Can you work these out from the model? Positions are in its coordinate system, mm. A direction names the side the tool comes from. Give positions to 0.01 mm unless a question says otherwise; leave off trailing zeros. Loops run counter-clockwise (first coordinate to the right, second up) from the corner with the lowest first, then second, coordinate; pieces in that order, holes last. Notation, with made-up numbers: (58, 79.5) - (79, 79.5) arc R13 ccw to (79, 83.5) - close; hole circle Ø8 at (88.5, 71). An arc over 180 degrees is marked (long way). Answer as a JSON object with one key per item and string values. Group by question number.
Item 1: Suppose I cut it at A-A on z = 77.5. Write out the boundary of the cut face in (x, y).
Item 2: Thinking about a two-plate mould opening in X: for faces 1 (the flat face through (-1, 1, 0)), 2 (the flat face through (27.978, -37, 5)), 3 (the flat face through (20, -37, 13)), 4 (the flat face through (-44, -1, 8)), which applies, pulls with the +X half, pulls with the -X half, needs draft (parallel to the pull), parting line crosses it, or undercut?
Item 3: Which directions (+Z, -Z, +X, -X, +Y, -Y) give clear straight access to the entire face, cutting with the end or side of a thin tool? Please do faces 5 (the cylindrical face through (-42, 14, 13)), 6 (the flat face through (21, -48.582, 5)), 7 (the flat face through (0, -58, 150)).
Item 4: Please list where these lines run through material, in increasing order: L1, parallel to Z at x = -6, y = 66; L2, parallel to X at y = -34, z = 49.5; L3, parallel to Y at x = -40, z = 77.
Item 5: Will these pins go through, and if not, where does the flat tip stop? pin 1 (1.5 mm diameter, centred on x = 22, z = -2, fed in from -Y); pin 2 (3 mm diameter, centred on x = -26.5, y = 0.5, fed in from -Z); pin 3 (8 mm diameter, centred on x = 17, y = -31.5, fed in from -Z).
Item 6: Suppose I cut it at B-B on y = 0. Write out the boundary of the cut face in (x, z).
Item 7: Suppose I cut it at C-C on x = 0. Write out the boundary of the cut face in (y, z), and give its area (3 significant figures).
Item 8: Suppose I cut it at D-D on x = -17. Write out the boundary of the cut face in (y, z), and give its area (3 significant figures).
from build123d import *

# Parameters (mm, degrees)
SKETCH_W        = 88
SKETCH_H        = 160
PAD_DEPTH       = 155
SKETCH001_R     = 66
POCKET_DEPTH    = 5
POCKET001_DEPTH = 5
SKETCH003_W     = 24
SKETCH003_H     = 31
PAD001_DEPTH    = 3
SKETCH004_W     = 16
SKETCH004_H     = 23
POCKET002_DEPTH = 16
CHAMFER_SIZE    = 3


with BuildPart() as part:
    # Sketch (on XY_Plane of Origin) → Pad (new body)
    with BuildSketch(Plane.XY):
        Rectangle(SKETCH_W, SKETCH_H)
    extrude(amount=PAD_DEPTH)

    # Sketch001 (on Face4 of Pad) → Pocket (cut)
    with BuildSketch(Plane(origin=(-44, 0, 0), x_dir=(0, -1, 0), z_dir=(-1, 0, 0))):
        with Locations((0, 77.5)):
            Circle(SKETCH001_R)
    extrude(amount=-POCKET_DEPTH, mode=Mode.SUBTRACT)

    # Sketch002 (on Face5 of Pocket) → Pocket001 (cut)
    with BuildSketch(Plane.XY.offset(155)):
        with BuildLine():
            ThreePointArc((20, -56.995285), (0, -36.995285), (-20, -56.995285))
            Line((-20, -56.995285), (-20, -80))
            Line((-20, -80), (20, -80))
            Line((20, -56.995285), (20, -80))
        make_face()
    extrude(amount=-POCKET001_DEPTH, mode=Mode.SUBTRACT)

    # Sketch003 (on Face2 of Pocket001) → Pad001 (join)
    with BuildSketch(Plane(origin=(0, 0, 0), x_dir=(1, 0, 0), z_dir=(0, 0, -1))):
        with Locations((19.978081, 37.081905)):
            Rectangle(SKETCH003_W, SKETCH003_H)
    extrude(amount=PAD001_DEPTH)

    # Sketch004 (on Face16 of Pad001) → Pocket002 (cut)
    with BuildSketch(Plane(origin=(0, 0, -3), x_dir=(1, 0, 0), z_dir=(0, 0, -1))):
        with Locations((19.978081, 37.081905)):
            Rectangle(SKETCH004_W, SKETCH004_H)
    extrude(amount=-POCKET002_DEPTH, mode=Mode.SUBTRACT)

    # Chamfer
    chamfer_edges = [part.edges().sort_by_distance(p)[0] for p in [
        (11.978081, -25.581905, 5),
        (11.978081, -48.581905, 5),
    ]]
    chamfer(chamfer_edges, length=CHAMFER_SIZE)


solid = part.part
Worked out:
{
 "1": {"outline": "(-44, -80) - (44, -80) - (44, 80) - (-44, 80) - (-44, 66) - (-39, 66) - (-39, -66) - (-44, -66) - close"},
 "2": {"face 1": "needs draft", "face 2": "undercut", "face 3": "undercut", "face 4": "pulls with the -X half"},
 "3": {"face 5": "-X", "face 6": "-Z", "face 7": "+Z, -Y"},
 "4": {"L1": "z = 0 to 155", "L2": "x = -39 to 44", "L3": "y = -80 to -66, 66 to 80"},
 "5": {"pin 1": "stops at y = -52.58", "pin 2": "stops at z = 0", "pin 3": "stops at z = 13"},
 "6": {"outline": "(-44, 0) - (44, 0) - (44, 155) - (-44, 155) - (-44, 143.5) - (-39, 143.5) - (-39, 11.5) - (-44, 11.5) - close"},
 "7": {"outline": "(-80, 0) - (80, 0) - (80, 155) - (-37, 155) - (-37, 150) - (-80, 150) - close", "area": "24,600 mm2"},
 "8": {"outline": "(-80, 0) - (80, 0) - (80, 155) - (-46.46, 155) - (-46.46, 150) - (-80, 150) - close", "area": "24,600 mm2"}
}
